Part print with two shaded views. Sizes in mm from the minimum x, y, z corner. Coordinates: 2 decimals unless noted, no trailing zeros. Order: outer loops, then holes, each group sorted by start corner. A loop starts at its lowest first (then second) coordinate and runs counter-clockwise, first axis right, second up. Notation, with made-up numbers: (9.5, 82.5) - (62.5, 82.5) arc R21 ccw to (62.5, 113.5) - close; hole circle Ø2 at (46, 53). An arc over 180 degrees is marked (long way). Write each question's results on one line, items separated by ' | '. Start each with the question number.
Q1. Band-saw the part on A-A, the plane x = 11.5. Write the cut outline in (y, z).
Q2. Band-saw the part on B-B, the plane z = 21.25. Write the cut outline in (x, y) (1 decimal), then the cut area to 3 significant figures.
Q3. Band-saw the part on C-C, the plane y = 17.75. Count the separate pieces of the cut face and the enclosed holes in it, then the cut area to 3 significant figures.
Q4. Pin check, flat tip, straight feed: P1, Ø3, axis at y = 4, z = 21.5, coming from the +X side. Stop position of the tip, or through.
Q5. Pull direction X, two halves, no side cores. Call the marked faces 1, 2, 3 and 4: released by +X, released by -X, zero draft, split by the parting line, or undercut.
Q6. Band-saw the part on D-D, the plane x = 17.25. Write the cut outline in (y, z).
Q7. Wall check: probe 1 along X at (y, z) = (16.75, 20.25) (1 decimal); probe 2 along Z at (x, y) = (11.25, 13); probe 3 along Z at (x, y) = (19, 21.75). Give the ranges that are in metal, low to high.
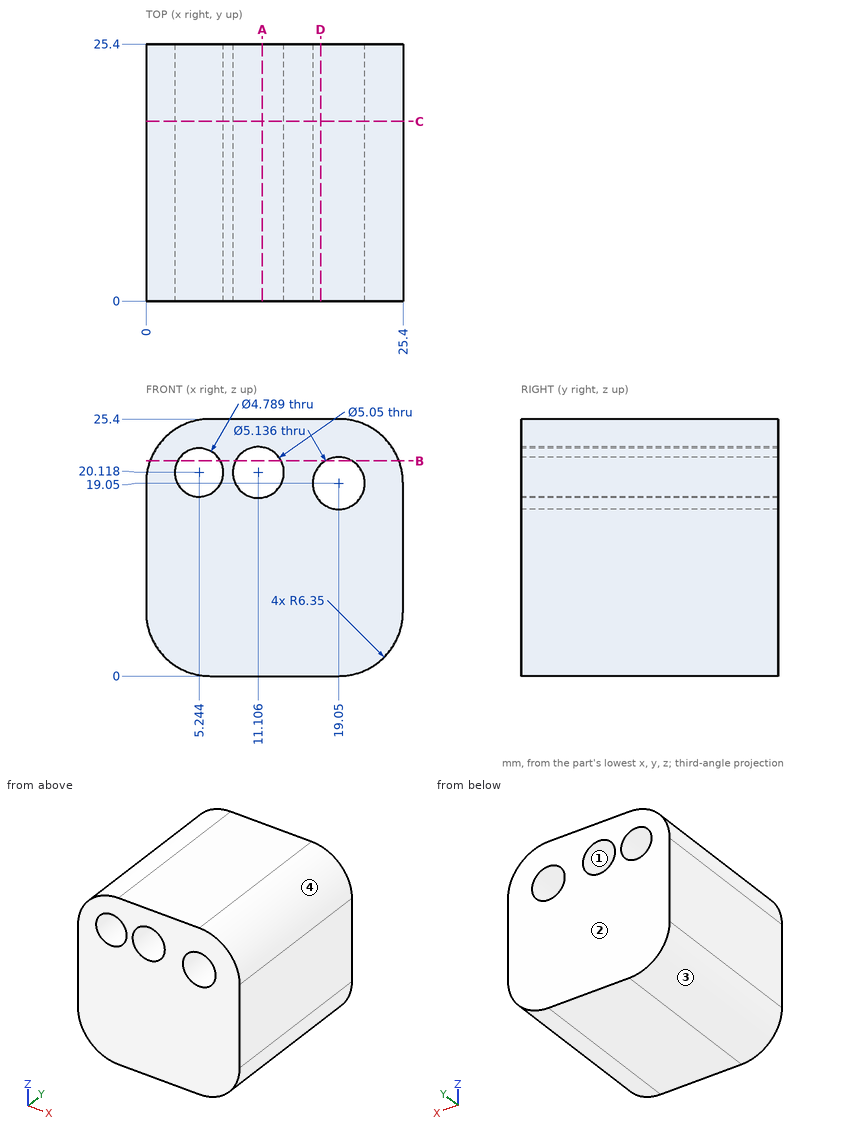
Results below:
1) outline: (0, 0) - (25.4, 0) - (25.4, 17.62) - (0, 17.62) - close; (0, 22.61) - (25.4, 22.61) - (25.4, 25.4) - (0, 25.4) - close
2) outline: (0.4, 0) - (3.1, 0) - (3.1, 25.4) - (0.4, 25.4) - close; (7.4, 0) - (8.8, 0) - (8.8, 25.4) - (7.4, 25.4) - close; (13.4, 0) - (17.7, 0) - (17.7, 25.4) - (13.4, 25.4) - close; (20.4, 0) - (25, 0) - (25, 25.4) - (20.4, 25.4) - close | area: 336 mm²
3) separate pieces: 1 | enclosed holes: 3 | area: 552 mm²
4) P1: stops at x = 25.33
5) face 1: undercut | face 2: zero draft | face 3: released by -X | face 4: released by +X
6) outline: (0, 0) - (25.4, 0) - (25.4, 17.22) - (0, 17.22) - close; (0, 20.88) - (25.4, 20.88) - (25.4, 25.4) - (0, 25.4) - close
7) probe 1: x = 0.1 to 2.9, 7.6 to 8.6, 13.6 to 16.8, 21.3 to 25.3 | probe 2: z = 0 to 17.6, 22.64 to 25.4 | probe 3: z = 0 to 16.48, 21.62 to 25.4
